Geometry: see drawing. Coordinates: mm, zero at the bounding-box minimum. A direction names the side the tool comes from. Give positions to 0.01 mm unless a question says otherwise; leave off trailing zeros. Loops run counter-clockwise (first coordinate to the right, second up) from the corner with the lowest first, then second, coordinate; pieces in that order, holes last. Notation, with made-up numbers: M 88,-5 L 142,-5 A12 cw 142,11 Z; hole C 61.5,46.25 d7. An arc over 180 degrees is marked long. Use a Markdown table: item, result. Add a question column.
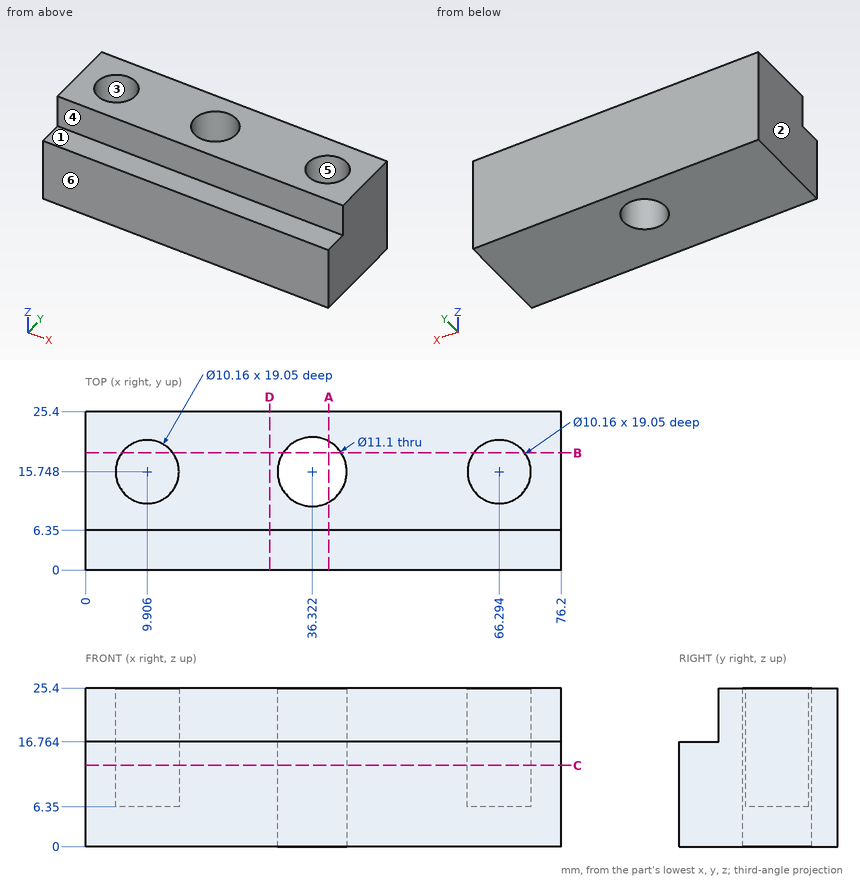
1) Contact query for flat-ended pins moving along their axis: P1, Ø5, axis at x = 8.5, y = 14, coming from the +Z side; P2, Ø3, axis at x = 35, y = 3, coming from the +Z side; P3, Ø7, axis at x = 43.5, z = 22.5, coming from the -Y side. Output: stop coordinate, or through.
2) Section query D-D, the plane x = 29.5. Return the cut outline in (y, z).
3) Section query C-C, the plane z = 13. Return the cut outline in (x, y).
4) Reachability of the marked faces 4, 5 and 6 from +Z, -Z, +X, -X, +Y, -Y: full face, straight path, thin tool, end or side. Return the list, or none.
5) Section query A-A, the plane x = 39. Return the cut outline in (y, z).
6) Ray query, line 1 (Z direction, x = 12.5, y = 5.75); line 2 (X direction, y = 18.25, z = 18.25) (1 decimal); line 3 (X direction, y = 20, z = 13.75) (1 decimal). Return the intervals inside material, ascending. Write a range as [from, to].
7) Section query B-B, the plane y = 18.75. Return the cut outline in (x, z).
8) Pull-direction query (X, two-part tool) for the marked faces 1, 2 and 3; classes: pulls with the +X half, pulls with the -X half, needs draft (parallel to the pull), parting line crosses it, or undercut.
Entries:
| question | item | result |
|---|---|---|
| 1 | P1 | stops at z = 6.35 |
| 1 | P2 | stops at z = 16.76 |
| 1 | P3 | stops at y = 6.35 |
| 2 | outline | M 0,0 L 25.4,0 L 25.4,25.4 L 6.35,25.4 L 6.35,16.76 L 0,16.76 Z |
| 3 | outline | M 0,0 L 76.2,0 L 76.2,25.4 L 0,25.4 Z; hole C 9.91,15.75 d10.16; hole C 36.32,15.75 d11.1; hole C 66.29,15.75 d10.16 |
| 4 | face 4 | +Z, +X, -X, -Y |
| 4 | face 5 | +Z |
| 4 | face 6 | +Z, -Z, +X, -X, -Y |
| 5 | outline | M 0,0 L 10.89,0 L 10.89,25.4 L 6.35,25.4 L 6.35,16.76 L 0,16.76 Z; M 20.61,0 L 25.4,0 L 25.4,25.4 L 20.61,25.4 Z |
| 6 | line 1 | z = [0, 16.76] |
| 6 | line 2 | x = [0, 5.5], [14.3, 31.4], [41.3, 61.9], [70.7, 76.2] |
| 6 | line 3 | x = [0, 7.1], [12.7, 32.8], [39.9, 63.5], [69.1, 76.2] |
| 7 | outline | M 0,0 L 31.65,0 L 31.65,25.4 L 14,25.4 L 14,6.35 L 5.81,6.35 L 5.81,25.4 L 0,25.4 Z; M 40.99,0 L 76.2,0 L 76.2,25.4 L 70.39,25.4 L 70.39,6.35 L 62.2,6.35 L 62.2,25.4 L 40.99,25.4 Z |
| 8 | face 1 | needs draft |
| 8 | face 2 | pulls with the -X half |
| 8 | face 3 | undercut |
